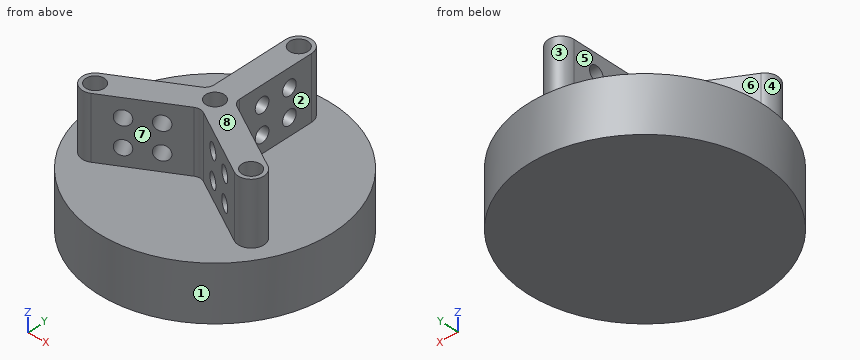
Autodesk Fusion 360 part; units mm, degrees
sketch "Sketch1" plane through (0, 0, 0) normal (0, 0, 1) x (1, 0, 0)
  line L0 (0, 0) -> (25, 0)
  line L1 (25, 0) -> (25, 48)
  line L2 (25, 48) -> (0, 48)
  line L3 (0, 48) -> (0, 0)
  dimension "d1" = 25
  dimension "d2" = 48
extrude "Extrude1" add sketch "Sketch1" along normal blind 15

Autodesk Fusion 360 part; units mm, degrees
sketch "Sketch1" plane through (0, 0, 0) normal (0, 0, 1) x (1, 0, 0)
  circle A0 centre (0, 0) radius 32
  circle A1 centre (0, 24.5) radius 2.5
  circle A2 centre (-21.2176, -12.25) radius 2.5
  circle A3 centre (21.2176, -12.25) radius 2.5
  circle A4 centre (0, 0) radius 2.5
  line L0 (-3.5, 3.4641) -> (-3.5, 24.5)
  line L1 (3.5, 24.5) -> (3.5, 3.4641)
  line L2 (-1.25, -4.7631) -> (-19.4676, -15.2811)
  line L3 (-22.9676, -9.2189) -> (-4.75, 1.299)
  line L4 (4.75, 1.299) -> (22.9676, -9.2189)
  line L5 (19.4676, -15.2811) -> (1.25, -4.7631)
  arc A5 (-4.75, 1.299) -> (-3.5, 3.4641) centre (-6, 3.4641) ccw
  arc A6 (3.5, 3.4641) -> (4.75, 1.299) centre (6, 3.4641) ccw
  arc A7 (1.25, -4.7631) -> (-1.25, -4.7631) centre (0, -6.9282) ccw
  arc A8 (3.5, 24.5) -> (-3.5, 24.5) centre (0, 24.5) ccw
  arc A9 (19.4676, -15.2811) -> (22.9676, -9.2189) centre (21.2176, -12.25) ccw
  arc A10 (-22.9676, -9.2189) -> (-19.4676, -15.2811) centre (-21.2176, -12.25) ccw
  dimension "d1" = 64
  dimension "d2" = 24.5
  dimension "d3" = 5
  dimension "d5" = 360
  dimension "d6" = 7
  dimension "d8" = 360
  dimension "d10" = 5
  dimension "d15" = 2.5
  dimension "d16" = 2.5
  dimension "d17" = 2.5
extrude "Extrude1" add sketch "Sketch1" along normal blind 32 contours L0 L1 L2 L3 L4 L5 A5 A6 A7 A8 A9 A10
sketch "Sketch2" plane through (1.75, -3.0311, 0) normal (0.5, -0.866, 0) x (0.866, 0.5, 0)
  line L0 (-24.5, 0) -> (-3.4641, 0)
  line L1 (-3.4641, 0) -> (-3.4641, 32)
  line L2 (-3.4641, 32) -> (-24.5, 32)
  line L3 (-24.5, 32) -> (-24.5, 0)
  line L4 (-24.5, 32) -> (-3.4641, 32)
  line L5 (-3.4641, 32) -> (-3.4641, 0)
  line L6 (-3.4641, 0) -> (-24.5, 0)
  line L7 (-24.5, 0) -> (-24.5, 32)
  circle A0 centre (-18, 27) radius 2
  circle A1 centre (-10, 27) radius 2
  circle A2 centre (-18, 19.6667) radius 2
  circle A3 centre (-10, 19.6667) radius 2
  circle A4 centre (-18, 12.3333) radius 2
  circle A5 centre (-10, 12.3333) radius 2
  circle A6 centre (-18, 5) radius 2
  circle A7 centre (-10, 5) radius 2
  dimension "d20" = 4
  dimension "d23" = 8
  dimension "d24" = -22
extrude "Extrude2" cut sketch "Sketch2" against normal blind 8 contours A0 | A1 | A2 | A3 | A4 | A5 | A6 | A7
pattern_circular "C-Pattern1" count 3 over 360 about axis through (0, 0, 1.75) along (0, 0, 1) of "Extrude2"
Geometry: final body of the model. Coordinates: model frame, mm. Face numbers are marked on the shaded views. A direction names the side the tool comes from. Give positions to 0.01 mm unless a question says otherwise; leave off trailing zeros. Loops run counter-clockwise (first coordinate to the right, second up) from the corner with the lowest first, then second, coordinate; pieces in that order, holes last. Notation, with made-up numbers: (42.25, -1.5) -> (76.25, -1.5) arc R24 ccw to (76.25, 29.5) -> close; hole circle Ø6 at (51, -20.75). An arc over 180 degrees is marked (long way). Return JSON: item names as keys, results as strings.
Item 1: Section A-A, the plane z = 16.5. Output: boundary loops of the cut face in (x, y).
Filled in:
{"outline": "(-22.97, -9.22) arc R3.5 ccw to (-19.47, -15.28) -> (-1.25, -4.76) arc R2.5 cw to (1.25, -4.76) -> (19.47, -15.28) arc R3.5 ccw to (22.97, -9.22) -> (4.75, 1.3) arc R2.5 cw to (3.5, 3.46) -> (3.5, 24.5) arc R3.5 ccw to (-3.5, 24.5) -> (-3.5, 3.46) arc R2.5 cw to (-4.75, 1.3) -> close; hole circle Ø5 at (-21.22, -12.25); hole circle Ø5 at (0, 0); hole circle Ø5 at (0, 24.5); hole circle Ø5 at (21.22, -12.25)"}
Item 2: Section B-B, the plane x = 0. Count the separate pieces of the cut face and the enclosed holes in it, plus the area to 3 significant figures.
Filled in:
{"separate pieces": "1", "enclosed holes": "8", "area": "1,240 mm^2"}
Item 3: Line query: line 1 (Y direction, x = 0, z = 22); line 2 (Z direction, x = -17, y = -9); line 3 (Z direction, x = 13, y = 20.5). Output: solid intervals per line, ascending.
Filled in:
{"line 1": "-4.43 to -2.5, 2.5 to 22, 27 to 28", "line 2": "0 to 3.42, 6.58 to 10.75, 13.92 to 18.08, 21.25 to 25.42, 28.58 to 32", "line 3": "0 to 15"}
Item 4: Pin query (flat end, axial travel): P1, Ø1.2, axis at y = 9.5, z = 13, coming from the -X side; P2, Ø1.5, axis at x = -22.5, z = 10, coming from the +Y side; P3, Ø2, axis at y = 11, z = 5.5, coming from the -X side. Return the tip coordinate at first contact, or that it passes through.
Filled in:
{"P1": "x = -30.74", "P2": "y = 23.47", "P3": "x = -30.4"}
Item 5: Mould query, pull axis X, two halves, no side actions, for the marked faces 6, 7 and 8. Classes: released by +X, released by -X, zero draft, split by the parting line, or undercut.
Filled in:
{"face 6": "released by -X", "face 7": "undercut", "face 8": "zero draft"}
Item 6: Access query for the marked faces 1, 2, 3, 4 and 5. Directions: +Z, -Z, +X, -X, +Y, -Y. A direction counts if a zero-diameter tool reaches every point of the face in a straight line with its end or side. Return the directions, or none.
Filled in:
{"face 1": "+Z, -Z", "face 2": "+Z, +X, +Y", "face 3": "+Z, +Y", "face 4": "+Z", "face 5": "+Z, -X, +Y"}
Item 7: Section D-D, the plane y = -24.5. Output: boundary loops of the cut face in (x, z).
Filled in:
{"outline": "(-20.59, 0) -> (20.59, 0) -> (20.59, 15) -> (-20.59, 15) -> close"}
